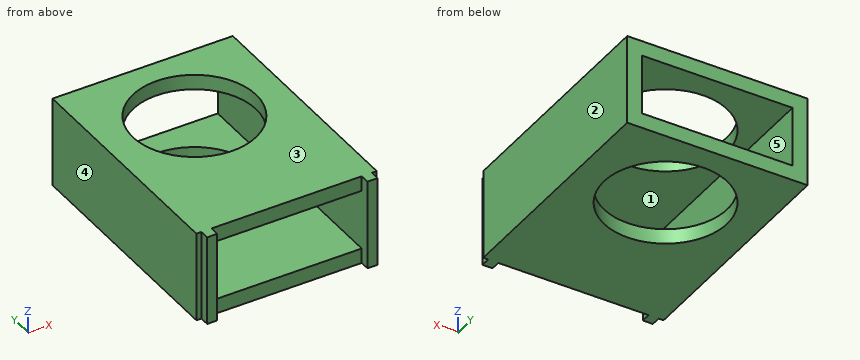
```python
from build123d import *

# Parameters (mm, degrees)
SKETCH2_W                = 38.1
SKETCH2_H                = 19.05
SKETCH2_W_2              = 31.75
SKETCH2_H_2              = 12.7
BOSS_EXTRUDE1_DEPTH      = 18
BOSS_EXTRUDE1_DEPTH_BACK = 32
SKETCH3_R                = 13
CUT_EXTRUDE1_DEPTH       = 20.05
SKETCH5_W                = 2.125
SKETCH5_H                = 19.05
BOSS_EXTRUDE2_DEPTH      = 2


with BuildPart() as part:
    # Sketch2 → Boss-Extrude1 (new body, two sides)
    with BuildSketch(Plane(origin=(0, 0, 0), x_dir=(1, 0, 0), z_dir=(0, 1, 0))) as boss_extrude1_sk:
        Rectangle(SKETCH2_W, SKETCH2_H)
        Rectangle(SKETCH2_W_2, SKETCH2_H_2, mode=Mode.SUBTRACT)
    extrude(amount=BOSS_EXTRUDE1_DEPTH)
    extrude(boss_extrude1_sk.sketch, amount=-BOSS_EXTRUDE1_DEPTH_BACK)

    # Sketch3 → Cut-Extrude1 (cut, through all)
    with BuildSketch(Plane.XY.offset(9.525)):
        Circle(SKETCH3_R)
    extrude(amount=-CUT_EXTRUDE1_DEPTH, mode=Mode.SUBTRACT)

    # Sketch5 → Boss-Extrude2 (add)
    with BuildSketch(Plane.XZ.offset(32)):
        with Locations((-16.9375, 0)):
            Rectangle(SKETCH5_W, SKETCH5_H)
        with Locations((16.9375, 0)):
            Rectangle(SKETCH5_W, SKETCH5_H)
    extrude(amount=BOSS_EXTRUDE2_DEPTH)


solid = part.part
```
Geometry check sheet. Reference: the model listing, model coordinates, mm. Face numbers are marked on the shaded views. A direction names the side the tool comes from. Give positions to 0.01 mm unless a question says otherwise; leave off trailing zeros. Order: outer loops, then holes, each group sorted by start corner. A loop starts at its lowest first (then second) coordinate and runs counter-clockwise, first axis right, second up.
1. Access from +Z, -Z, +X, -X, +Y, -Y to the whole of each face (thin tool, end or side, straight path). Record for the marked faces 1 and 2.
2. Section check D-D, the plane y = -27. Enter the section's corners in (x, z) (3 decimals), and give its area (3 significant figures).
3. Release check for a two-part mould opening along Z. For the marked faces 3, 4 and 5 record: pulls with the +Z half, pulls with the -Z half, needs draft (parallel to the pull), parting line crosses it, or undercut.
4. Section check A-A, the plane x = 0. Enter the section's corners in (y, z) (3 decimals).
5. Section check B-B, the plane y = 0. Enter the section's corners in (x, z) (3 decimals).
6. Thickness scan on L1, parallel to X at y = 14, z = 0.5 (3 decimals); L2, parallel to Z at x = -11, y = -25.5 (3 decimals); L3, parallel to Y at x = 0, z = 8.85. Record the ranges inside material, lowest first.
7. Gauge pin test, flat ends, axial feed: pin 1 Ø1 at (x, z) = (-3.5, -7.5) entering from -Y; pin 2 Ø8 at (x, y) = (9.5, -6) entering from -Z (3 decimals); pin 3 Ø6 at (x, z) = (-6, -1) entering from -Y; pin 4 Ø1.6 at (y, z) = (-33, 1.5) entering from +X. Record the tip position at first contact, or that the pin passes through.
8. Section check C-C, the plane z = -2. Enter the section's corners in (x, y) (3 decimals), and give its area (3 significant figures).
Values follow:
1. face 1: +Y, -Y
1. face 2: +Z, -Z, +X, +Y, -Y
2. outline: (-19.05, -9.525) - (19.05, -9.525) - (19.05, 9.525) - (-19.05, 9.525) - close; hole (-15.875, -6.35) - (15.875, -6.35) - (15.875, 6.35) - (-15.875, 6.35) - close
2. area: 323 mm2
3. face 3: pulls with the +Z half
3. face 4: needs draft
3. face 5: undercut
4. outline: (-32, -9.525) - (-13, -9.525) - (-13, -6.35) - (-32, -6.35) - close; (-32, 6.35) - (-13, 6.35) - (-13, 9.525) - (-32, 9.525) - close; (13, -9.525) - (18, -9.525) - (18, -6.35) - (13, -6.35) - close; (13, 6.35) - (18, 6.35) - (18, 9.525) - (13, 9.525) - close
5. outline: (-19.05, -9.525) - (-13, -9.525) - (-13, -6.35) - (-15.875, -6.35) - (-15.875, 6.35) - (-13, 6.35) - (-13, 9.525) - (-19.05, 9.525) - close; (13, -9.525) - (19.05, -9.525) - (19.05, 9.525) - (13, 9.525) - (13, 6.35) - (15.875, 6.35) - (15.875, -6.35) - (13, -6.35) - close
6. L1: x = -19.05 to -15.875, 15.875 to 19.05
6. L2: z = -9.525 to -6.35, 6.35 to 9.525
6. L3: y = -32 to -13, 13 to 18
7. pin 1: stops at y = -32
7. pin 2: stops at z = -9.525
7. pin 3: passes through
7. pin 4: stops at x = 18
8. outline: (-19.05, -32) - (-18, -32) - (-18, -34) - (-15.875, -34) - (-15.875, 18) - (-19.05, 18) - close; (15.875, -34) - (18, -34) - (18, -32) - (19.05, -32) - (19.05, 18) - (15.875, 18) - close
8. area: 326 mm2
